Read the model definition and answer for the solid it produces. Units are mm, in the model's axes. Face numbers are marked on the shaded views. A direction names the side the tool comes from. Coordinates: 2 decimals unless noted, no trailing zeros. Loops run counter-clockwise (first coordinate to the right, second up) from the corner with the lowest first, then second, coordinate; pieces in that order, holes last. Notation, with made-up numbers: (11.5, -19.75) - (15.5, -19.75) arc R29 ccw to (15.5, 5.25) - close; hole circle Ø11 at (25, 43.5). An arc over 180 degrees is marked (long way). Use one line per item in the form item = value.
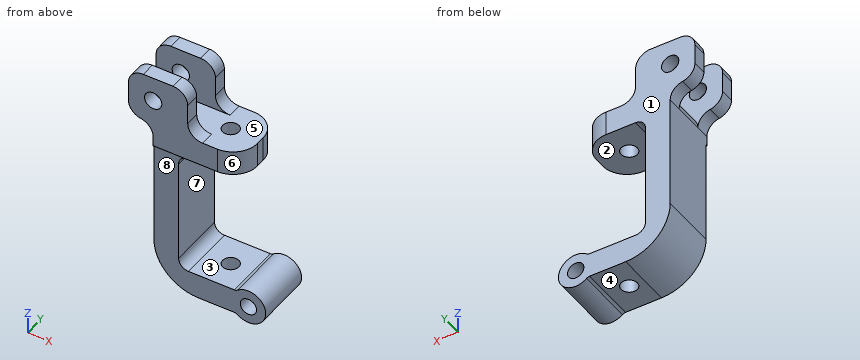
from build123d import *

# Parameters (mm, degrees)
SKETCH1_W               = 20.25
SKETCH1_H               = 11.5
BOSS_EXTRUDE1_DEPTH     = 5
SKETCH2_W               = 5
SKETCH2_H               = 11.5
BOSS_EXTRUDE2_DEPTH     = 25
SKETCH3_W               = 18
SKETCH3_H               = 11.75
BOSS_EXTRUDE3_DEPTH     = 5
CUT_EXTRUDE2_DEPTH      = 33.226008518
CUT_EXTRUDE2_DEPTH_BACK = 33.226008518
SKETCH5_R               = 1.65
FILLET1_R               = 9
FILLET7_R               = 5
CUT_EXTRUDE4_DEPTH      = 39.206879289
CUT_EXTRUDE4_DEPTH_BACK = 39.206879289
SKETCH10_R              = 1.65
SKETCH10_4_R            = 3.5
SKETCH10_4_R_2          = 1.65
BOSS_EXTRUDE7_DEPTH     = 11.5
FILLET13_R              = 1
FILLET16_R              = 2
SKETCH11_W              = 12
SKETCH11_H              = 2.875
BOSS_EXTRUDE8_DEPTH     = 10
CUT_EXTRUDE5_DEPTH      = 49.906319888
CUT_EXTRUDE5_DEPTH_BACK = 49.906319888
SKETCH12_R              = 1.75
FILLET17_R              = 3
FILLET18_R              = 3
FILLET19_R              = 3
FILLET20_R              = 2


with BuildPart() as part:
    # Sketch1 → Boss-Extrude1 (new body)
    with BuildSketch(Plane.XY):
        Rectangle(SKETCH1_W, SKETCH1_H)
    extrude(amount=BOSS_EXTRUDE1_DEPTH)

    # Sketch2 → Boss-Extrude2 (add)
    with BuildSketch(Plane.XY.offset(5)):
        with Locations((-7.625, 0)):
            Rectangle(SKETCH2_W, SKETCH2_H)
    extrude(amount=BOSS_EXTRUDE2_DEPTH)

    # Sketch3 → Boss-Extrude3 (add)
    with BuildSketch(Plane.XY.offset(30)):
        with Locations((-1.125, -0.125)):
            Rectangle(SKETCH3_W, SKETCH3_H)
    extrude(amount=BOSS_EXTRUDE3_DEPTH)

    # Sketch5 → Cut-Extrude2 (cut, two sides: drawn at the far end of the back side and taken through both)
    with BuildSketch(Plane(origin=(0, 0, 30), x_dir=(-1, 0, 0), z_dir=(0, 0, -1)).offset(-CUT_EXTRUDE2_DEPTH_BACK)):
        with Locations((-1.875, -0.125)):
            Circle(SKETCH5_R)
    extrude(amount=CUT_EXTRUDE2_DEPTH + CUT_EXTRUDE2_DEPTH_BACK, mode=Mode.SUBTRACT)

    # Fillet1
    fillet1_edges = [part.edges().sort_by_distance(p)[0] for p in [
        (-10.125, 0, 0),
    ]]
    fillet(fillet1_edges, radius=FILLET1_R)

    # Fillet7
    fillet7_edges = [part.edges().sort_by_distance(p)[0] for p in [
        (7.875, -6, 32.5),
        (7.875, 5.75, 32.5),
    ]]
    fillet(fillet7_edges, radius=FILLET7_R)

    # Sketch10 → Cut-Extrude4 (cut, two sides: drawn at the far end of the back side and taken through both)
    with BuildSketch(Plane.XZ.offset(5.75).offset(-CUT_EXTRUDE4_DEPTH_BACK)):
        with Locations((9, 2.5)):
            Circle(SKETCH10_R)
    extrude(amount=CUT_EXTRUDE4_DEPTH + CUT_EXTRUDE4_DEPTH_BACK, mode=Mode.SUBTRACT)

    # Sketch10_4 → Boss-Extrude7 (add)
    with BuildSketch(Plane.XZ.offset(5.75)):
        with Locations((9, 2.5)):
            Circle(SKETCH10_4_R)
        with Locations(Location((9, 2.5, 0), (0, 0, 270))):
            Circle(SKETCH10_4_R_2, mode=Mode.SUBTRACT)
    extrude(amount=-BOSS_EXTRUDE7_DEPTH)

    # Fillet13
    fillet13_edges = [part.edges().sort_by_distance(p)[0] for p in [
        (6.550510257, 0, 0),
        (6.550510257, 0, 5),
    ]]
    fillet(fillet13_edges, radius=FILLET13_R)

    # Fillet16
    fillet16_edges = [part.edges().sort_by_distance(p)[0] for p in [
        (-5.125, 0, 5),
    ]]
    fillet(fillet16_edges, radius=FILLET16_R)

    # Sketch11 → Boss-Extrude8 (add)
    with BuildSketch(Plane.XY.offset(35)):
        with Locations((-9.125, 4.3125)):
            Rectangle(SKETCH11_W, SKETCH11_H)
        with Locations((-9.125, -4.5625)):
            Rectangle(SKETCH11_W, SKETCH11_H)
    extrude(amount=BOSS_EXTRUDE8_DEPTH)

    # Sketch12 → Cut-Extrude5 (cut, two sides: drawn at the far end of the back side and taken through both)
    with BuildSketch(Plane(origin=(0, 5.75, 0), x_dir=(1, 0, 0), z_dir=(0, 1, 0)).offset(-CUT_EXTRUDE5_DEPTH_BACK)):
        with Locations(Location((-10.125, -40, 0), (0, 0, 90))):
            Circle(SKETCH12_R)
    extrude(amount=CUT_EXTRUDE5_DEPTH + CUT_EXTRUDE5_DEPTH_BACK, mode=Mode.SUBTRACT)

    # Fillet17
    fillet17_edges = [part.edges().sort_by_distance(p)[0] for p in [
        (-10.125, -4.5625, 35),
        (-15.125, 4.3125, 45),
        (-3.125, 4.3125, 35),
        (-3.125, 4.3125, 45),
        (-3.125, -4.5625, 35),
        (-3.125, -4.5625, 45),
        (-15.125, -4.5625, 45),
        (-10.125, 4.3125, 35),
    ]]
    fillet(fillet17_edges, radius=FILLET17_R)

    # Fillet18
    fillet18_edges = [part.edges().sort_by_distance(p)[0] for p in [
        (-15.125, 4.3125, 35),
        (-15.125, -4.5625, 35),
    ]]
    fillet(fillet18_edges, radius=FILLET18_R)

    # Fillet19
    fillet19_edges = [part.edges().sort_by_distance(p)[0] for p in [
        (-10.125, -0.125, 35),
    ]]
    fillet(fillet19_edges, radius=FILLET19_R)

    # Fillet20
    fillet20_edges = [part.edges().sort_by_distance(p)[0] for p in [
        (-5.125, 0, 30),
    ]]
    fillet(fillet20_edges, radius=FILLET20_R)


solid = part.part
Item 1: Each of these flat-tipped pins is pushed along its axis until it touches: P1, Ø3, axis at x = 1.875, y = -0.125, coming from the +Z side; P2, Ø2, axis at y = 1, z = 26, coming from the +X side (3 decimals); P3, Ø10, axis at x = -5, z = 6, coming from the -Y side; P4, Ø4.5, axis at x = 1.875, y = -0.125, coming from the -Z side. Where does it stop, or does it pass through?
Results below:
P1 = through
P2 = -5.125
P3 = -5.75
P4 = 0
Item 2: The part is cut by section C-C on x = 9. Give the vertices of the cut face in (y, z), plus the area to 4 significant figures.
Results below:
outline = (-5.75, -1) - (5.75, -1) - (5.75, 0.85) - (-5.75, 0.85) - close; (-5.75, 4.15) - (5.75, 4.15) - (5.75, 6) - (-5.75, 6) - close
area = 42.55 mm²
Item 3: The part is cut by section D-D on x = -10.75. Give the vertices of the cut face in (y, z) (3 decimals).
Results below:
outline = (-6, 33.833) - (-3.125, 33.833) - (-3.125, 38.365) - (-6, 38.365) - close; (-6, 41.635) - (-3.125, 41.635) - (-3.125, 45) - (-6, 45) - close; (2.875, 33.833) - (5.75, 33.833) - (5.75, 38.365) - (2.875, 38.365) - close; (2.875, 41.635) - (5.75, 41.635) - (5.75, 45) - (2.875, 45) - close
Item 4: Find the intervals of material crossed by L1, parallel to X at y = -4.4, z = 40 (3 decimals); L2, parallel to Z at x = 9, y = -5; L3, parallel to Z at x = -0.5, y = 0, in increasing order.
Results below:
L1 = -15.125 to -11.875, -8.375 to -3.125
L2 = -1 to 0.85, 4.15 to 6
L3 = 0 to 5, 30 to 35
Item 5: For a pull along Z with two mould halves and no side action, classify the marked faces 1, 2, 3 and 4 as +Z half, -Z half, draft (parallel to the pull), parting line (faces both ways), or undercut.
Results below:
face_1 = draft
face_2 = undercut
face_3 = undercut
face_4 = -Z half
Item 6: The part is cut by section A-A on z = 40. Give the vertices of the cut face in (x, y) (3 decimals).
Results below:
outline = (-15.125, -6) - (-11.875, -6) - (-11.875, -3.125) - (-15.125, -3.125) - close; (-15.125, 2.875) - (-11.875, 2.875) - (-11.875, 5.75) - (-15.125, 5.75) - close; (-8.375, -6) - (-3.125, -6) - (-3.125, -3.125) - (-8.375, -3.125) - close; (-8.375, 2.875) - (-3.125, 2.875) - (-3.125, 5.75) - (-8.375, 5.75) - close
Item 7: The part is cut by section B-B on z = 2.5. Give the vertices of the cut face in (x, y) (3 decimals), plus the area to 3 significant figures.
Results below:
outline = (-7.35, -5.75) - (7.35, -5.75) - (7.35, 5.75) - (-7.35, 5.75) - close; (10.65, -5.75) - (12.5, -5.75) - (12.5, 5.75) - (10.65, 5.75) - close; hole circle Ø3.3 at (1.875, -0.125)
area = 182 mm²
Item 8: Which of the six approach directions +Z, -Z, +X, -X, +Y, -Y give full straight-line access (tool end or side, diameter ignored) to the marked faces 5, 6, 7 and 8?
Results below:
face_5 = +Z, +X
face_6 = +Z, +X, -Y
face_7 = +X, +Y, -Y
face_8 = -Z, +X, -X, -Y
